Could you check a few things on this model? Use its own coordinates, in mm. Coordinates: 2 decimals unless noted, no trailing zeros. Order: outer loops, then holes, each group sorted by start corner. A loop starts at its lowest first (then second) coordinate and runs counter-clockwise, first axis right, second up. Notation, with made-up numbers: (87, 40.5) -> (142, 40.5) arc R24 ccw to (142, 61.5) -> close; hole circle Ø4 at (-18, 54). An arc over 180 degrees is marked (long way). Put each result on its own line as item: value. Start each with the question number.
Q1. If we section it at A-A (y = 1.5): Please give me the cut outline in (x, z), and give its area (3 significant figures).
Q2. If we section it at B-B (z = -162): Please give me the cut outline in (x, y), and give its area (3 significant figures).
Q3. Please list where these lines run through material, in increasing order: line 1 along Z through (x, y) = (-22, 2.1); line 2 along X through (y, z) = (2.75, -163); line 3 along Z through (x, y) = (-85, 0.65).
Q4. Will these pins go through, and if not, where does the flat tip stop? pin 1 (0.7 mm diameter, centred on x = -3.5, y = 2.5, fed in from -Z); pin 2 (2.5 mm diameter, centred on y = 2, z = -171.5, fed in from +X); pin 3 (2 mm diameter, centred on y = 4, z = -56.5, fed in from +X).
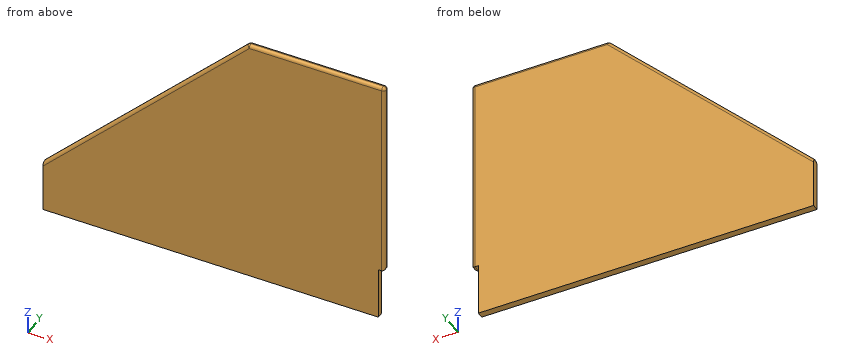
from build123d import *

# Parameters (mm, degrees)
BOSS_EXTRUDE2_DEPTH = 4.76
FILLET11_R          = 2.38


with BuildPart() as part:
    # Sketch1 → Boss-Extrude2 (new body)
    with BuildSketch(Plane(origin=(0, 0, 0), x_dir=(1, 0, 0), z_dir=(0, 1, 0))):
        Polygon((0, 0), (0, 150), (-4.8006, 150), (-4.8006, 188.989), (-249.8006, 188.989), (-249.8006, 150), (-99.9998, 0), align=None)
    extrude(amount=BOSS_EXTRUDE2_DEPTH)

    # Fillet11
    fillet11_edges = [part.edges().sort_by_distance(p)[0] for p in [
        (-49.9999, 0, 0),
        (-99.9998, 2.38, 0),
        (-249.8006, 2.38, -150),
        (0, 2.38, -150),
        (0, 2.38, 0),
        (-174.9002, 4.76, -75),
        (-49.9999, 4.76, 0),
        (-174.9002, 0, -75),
        (0, 4.76, -75),
        (0, 0, -75),
    ]]
    fillet(fillet11_edges, radius=FILLET11_R - 0.0001)  # a hair under: the kernel refuses the full size


solid = part.part
The answers:
1. outline: (-249.8, -188.99) -> (-4.8, -188.99) -> (-4.8, -150) -> (-2.38, -150) arc R2.38 ccw to (-0.17, -148.5) -> (-0.17, -2.38) arc R2.21 ccw to (-2.38, -0.17) -> (-99.01, -0.17) arc R2.21 ccw to (-100.58, -0.82) -> (-249.61, -150.04) arc R2.38 ccw to (-249.8, -150.98) -> close
1. area: 35,700 mm^2
2. outline: (-249.8, 0) -> (-4.8, 0) -> (-4.8, 4.76) -> (-249.8, 4.76) -> close
2. area: 1,170 mm^2
3. line 1: -188.99 to -0.02
3. line 2: -249.8 to -4.8
3. line 3: -188.99 to -0.75
4. pin 1: z = -150
4. pin 2: x = -4.8
4. pin 3: x = -0.08
